Autodesk Inventor part; units mm, degrees
ref_plane "Work Plane2" through (28.3083, 0, 0) normal (1, 0, 0) x (0, 1, 0)
ref_plane "XZ Plane" through (0, 0, 0) normal (0, 1, 0) x (-1, 0, 0)
ref_plane "XY Plane" through (0, 0, 0) normal (0, 0, 1) x (1, 0, 0)
sketch "Sketch1" plane through (0, 0, 0) normal (0, 0, 1) x (1, 0, 0)
  line L0 (0, 0) -> (56.6166, 0)
  line L1 (56.6166, 0) -> (56.6166, 56.6166)
  line L2 (56.6166, 56.6166) -> (0, 56.6166)
  line L3 (0, 56.6166) -> (0, 0)
  circle A0 centre (28.3083, 56.6166) radius 1.75
  circle A1 centre (28.3083, 56.6166) radius 6.35
  arc A2 (0, 0) -> (21.9587, 56.6898) centre (-64.7797, 57.6901) ccw
  arc A3 (6.3496, 0) -> (25.2456, 34.8225) centre (-58.4301, 57.6901) ccw
  line L4 (28.3083, 0) -> (28.3083, 56.6898)
  arc A4 (34.6579, 56.6898) -> (56.6166, 0) centre (121.3963, 57.6901) ccw
  arc A5 (31.371, 34.8225) -> (50.267, 0) centre (115.0467, 57.6901) ccw
  arc A6 (31.371, 34.8225) -> (25.2456, 34.8225) centre (28.3083, 33.9855) ccw
  point P0 (21.9583, 56.6166)
  point P1 (21.9578, 56.6166)
  point P2 (6.3496, 0)
  point P3 (50.267, 0)
  point P4 (34.6588, 56.6166)
  point P5 (34.6583, 56.6166)
  dimension "d3" = 12.7
  dimension "d0" = 56.6166
  dimension "d1" = 56.6166
  dimension "d2" = 3.5
  dimension "d4" = 3.175
extrude "Extrusion1" add sketch "Sketch1" along normal blind 9.525 contours A2 A1 L4 A6 A3 L0 | A1 L2 A0 | L2 A0 L4 A1 | L4 A0 L2 A1 | A1 A4 L0 A5 A6 L4
ref_plane "Work Plane2" through (28.3083, 0, 0) normal (1, 0, 0) x (0, 1, 0)
ref_plane "Work Plane1" through (56.6166, 0, 0) normal (1, 0, 0) x (0, 1, 0)
properties part number "transfer gear rod support end"
Design review of the part built by this model. Coordinates are the model's own, in mm. A direction names the side the tool comes from. Give positions to 0.01 mm unless a question says otherwise; leave off trailing zeros. Loops run counter-clockwise (first coordinate to the right, second up) from the corner with the lowest first, then second, coordinate; pieces in that order, holes last. Notation, with made-up numbers: (77.25, -6) -> (118.25, -6) arc R7 ccw to (118.25, 5) -> close; hole circle Ø3 at (84.5, 20.5). An arc over 180 degrees is marked (long way). One line per question, with ' | ' between items. Start each with the question number.
(1) For faces 1 (the face through (38.94, 16.07, 4.7)), 2 (the face through (16.25, 26.73, 4.7)), list the 3-axis set-ups (+Z, -Z, +X, -X, +Y, -Y) from which the entire face can be reached by the end or side of a thin tool; tool diameter is ignored.
(2) Insertion check: P1, Ø8, axis at x = 41, y = 40, coming from the +Z side; P2, Ø3, axis at x = 23.5, y = 26, coming from the +Z side (3 decimals). Each pin has a flat end and moves straight along its axis. Give the tip position at first contact, or say it passes through.
(3) We need section B-B (z = 4.75). State the section outline as (x, y) points.
(4) We need section A-A (y = 57.5). State the section outline as (x, z) points (3 decimals).
(5) We need section C-C (y = 33). State the section outline as (x, z) points (1 decimal), and give its area (3 significant figures).
(6) For line 1 (X direction, y = 36, z = 2.5); line 2 (X direction, y = 32.5, z = 7.25); line 3 (Y direction, x = 9, z = 3.5), list the stretches that pass through material, from the lowest coordinate up.
(7) We need section D-D (x = 13). State the section outline as (y, z) points (3 decimals).
The answers:
1) face 1: +Z, -Z, -Y | face 2: +Z, -Z, -X, +Y
2) P1: passes through | P2: stops at z = 9.525
3) outline: (0, 0) -> (6.35, 0) arc R86.74 ccw to (25.25, 34.82) arc R3.18 cw to (31.37, 34.82) arc R86.74 ccw to (50.27, 0) -> (56.62, 0) arc R86.74 cw to (34.66, 56.62) arc R6.35 ccw to (21.96, 56.62) arc R86.74 cw to start; hole circle Ø3.5 at (28.31, 56.62)
4) outline: (22.02, 0) -> (26.798, 0) -> (26.798, 9.525) -> (22.02, 9.525) -> close; (29.819, 0) -> (34.597, 0) -> (34.597, 9.525) -> (29.819, 9.525) -> close
5) outline: (18.4, 0) -> (24.7, 0) -> (24.7, 9.5) -> (18.4, 9.5) -> close; (31.9, 0) -> (38.2, 0) -> (38.2, 9.5) -> (31.9, 9.5) -> close | area: 121 mm^2
6) line 1: x = 19.21 to 25.85, 30.76 to 37.41 | line 2: x = 18.23 to 24.58, 32.04 to 38.39 | line 3: y = 3.12 to 12.07
7) outline: (8.473, 0) -> (19.286, 0) -> (19.286, 9.525) -> (8.473, 9.525) -> close
